```python
from build123d import *

# Parameters (mm, degrees)
SKETCH2_W                                     = 42.8625
SKETCH2_H                                     = 7.9375
BOSS_EXTRUDE1_DEPTH                           = 1.8034
SKETCH3_W                                     = 10.16
SKETCH3_H                                     = 7.9375
BOSS_EXTRUDE2_DEPTH                           = 7.62
CUT_EXTRUDE1_DEPTH                            = 35.69005
CSK_FOR_6_FLAT_HEAD_MACHINE_SCREW1_AT_2_COUNT = 2
CSK_FOR_6_FLAT_HEAD_MACHINE_SCREW1_AT_2_PITCH = 34.52812501


with BuildPart() as part:
    # Sketch2 → Boss-Extrude1 (new body)
    with BuildSketch(Plane(origin=(0, 0, 0), x_dir=(1, 0, 0), z_dir=(0, 1, 0))):
        with Locations((-21.724415377, -11.319579887)):
            Rectangle(SKETCH2_W, SKETCH2_H)
    extrude(amount=BOSS_EXTRUDE1_DEPTH)

    # Sketch3 → Boss-Extrude2 (add)
    with BuildSketch(Plane(origin=(0, 1.8034, 0), x_dir=(1, 0, 0), z_dir=(0, 1, 0))):
        with Locations((-29.903215377, -11.319579887)):
            Rectangle(SKETCH3_W, SKETCH3_H)
        with Locations((-13.545615377, -11.319579887)):
            Rectangle(SKETCH3_W, SKETCH3_H)
    extrude(amount=BOSS_EXTRUDE2_DEPTH)

    # Sketch5 → Cut-Extrude1 (cut, through all)
    with BuildSketch(Plane.ZY.offset(34.983215377)):
        with BuildLine():
            Line((7.350829887, 8.005737457), (7.350829887, 10.117841345))
            Line((7.350829887, 10.117841345), (15.288329887, 10.117841345))
            Line((15.288329887, 10.117841345), (15.288329887, 8.005737457))
            ThreePointArc((15.288329887, 8.005737457), (11.319579887, 9.459221838), (7.350829887, 8.005737457))
        make_face()
    extrude(amount=-CUT_EXTRUDE1_DEPTH, mode=Mode.SUBTRACT)

    # Sketch6 → CSK for #6 Flat Head Machine Screw1 (revolve, cut)
    with BuildSketch(Plane(origin=(-4.460352877, 1.8034, 11.319579887), x_dir=(0, 0, 1), z_dir=(1, 0, 0))):
        Polygon((0, 0), (0, 1.8034), (1.89865, 1.8034), (1.89865, 1.891953401), (3.5433, 0), align=None)
    csk_for_6_flat_head_machine_screw1 = revolve(axis=Axis((-4.460352877, 8.1534, 11.319579887), (0, -1, 0)), mode=Mode.SUBTRACT)

    # CSK for #6 Flat Head Machine Screw1 at 2: CSK for #6 Flat Head Machine Screw1 ×2
    with Locations(*[(-i * CSK_FOR_6_FLAT_HEAD_MACHINE_SCREW1_AT_2_PITCH, 0, 0) for i in range(1, CSK_FOR_6_FLAT_HEAD_MACHINE_SCREW1_AT_2_COUNT)]):
        add(csk_for_6_flat_head_machine_screw1, mode=Mode.SUBTRACT)


solid = part.part
```
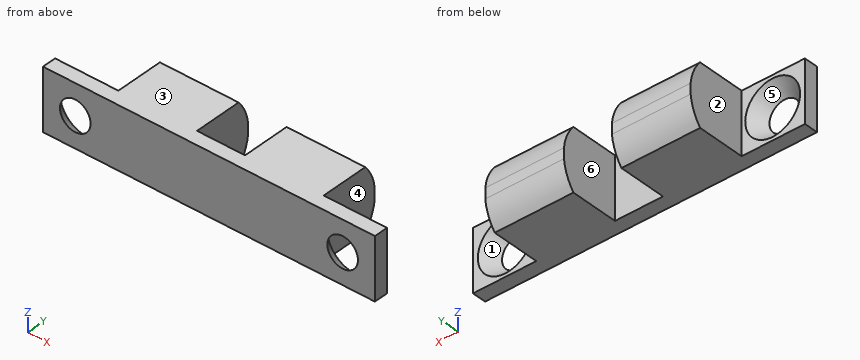
Read the model definition and answer for the solid it produces. Units are mm, in the model's axes. Face numbers are marked on the shaded views. A direction names the side the tool comes from. Give positions to 0.01 mm unless a question says otherwise; leave off trailing zeros. Order: outer loops, then holes, each group sorted by start corner. A loop starts at its lowest first (then second) coordinate and runs counter-clockwise, first axis right, second up. Notation, with made-up numbers: (44.5, -25) -> (53.5, -25) arc R26 cw to (53.5, 0) -> close; hole circle Ø9 at (57, 36). An arc over 180 degrees is marked (long way). One line per item, written item: value. Start each with the question number.
(1) The part is cut by section A-A (y = 4.5). Determine the outline of the cut face in (x, z), and give its area (3 significant figures).
(2) The part is cut by section B-B (x = -33). Determine the outline of the cut face in (y, z), and give its area (3 significant figures).
(3) Straight lines are drawn through the part: L1, parallel to X at y = 3.75, z = 9.75; L2, parallel to X at y = 0.75, z = 10; L3, parallel to X at y = 1.25, z = 13. For each, find the intervals that lie inside material, in ascending order.
(4) The part is cut by section C-C (y = 1). Determine the outline of the cut face in (x, z), and give its area (3 significant figures).
(5) For a pull along X with two mould halves and no side action, classify the marked faces 1, 2, 3 and 4 as released by +X, released by -X, zero draft, split by the parting line, or undercut.
(6) Flat-ended cylindrical pins translate along their axes: P1, Ø4, axis at x = -10.5, z = 13, coming from the -Y side; P2, Ø3, axis at x = -23, z = 10, coming from the +Y side; P3, Ø2.5, axis at y = 6, z = 11, coming from the -X side. Find the tip coordinate at first contact, or state that the pin passes through.
(7) The part is cut by section D-D (z = 10). State how many separate pieces and enclosed holes the cut face has, and give its area (3 significant figures).
(8) A tool of negligible diameter and unlimited length cuts with its end or side. For the marked faces 5 and 6, from which of +Z, -Z, +X, -X, +Y, -Y can it reach the whole face along a straight path? Write none if from no direction.
Taken from the geometry:
1. outline: (-34.98, 7.35) -> (-24.82, 7.35) -> (-24.82, 15.29) -> (-34.98, 15.29) -> close; (-18.63, 7.35) -> (-8.47, 7.35) -> (-8.47, 15.29) -> (-18.63, 15.29) -> close
1. area: 161 mm^2
2. outline: (0, 7.35) -> (8.01, 7.35) arc R6.15 ccw to (9.42, 10.66) -> (9.42, 11.98) arc R6.15 ccw to (8.01, 15.29) -> (0, 15.29) -> close
2. area: 71.4 mm^2
3. L1: -34.98 to -24.82, -18.63 to -8.47
3. L2: -43.16 to -41.26, -36.72 to -6.73, -2.19 to -0.29
3. L3: -43.16 to -41.55, -36.43 to -7.02, -1.9 to -0.29
4. outline: (-43.16, 7.35) -> (-0.29, 7.35) -> (-0.29, 15.29) -> (-43.16, 15.29) -> close; hole circle Ø5.69 at (-38.99, 11.32); hole circle Ø5.69 at (-4.46, 11.32)
4. area: 289 mm^2
5. face 1: undercut
5. face 2: released by -X
5. face 3: zero draft
5. face 4: released by +X
6. P1: y = 0
6. P2: y = 1.8
6. P3: x = -34.98
7. separate pieces: 3
7. enclosed holes: 0
7. area: 213 mm^2
8. face 5: +Y
8. face 6: +Z, -Z, +Y
